```python
from build123d import *

# Parameters (mm, degrees)
F1_DEPTH = 2


with BuildPart() as f1:
    # F0 (on Top) → F1 (new body)
    with BuildSketch(Plane.XY):
        Polygon((0, 10), (0, 0), (10, 0), (300, 0), (300, 10), (10, 10), (10, 300), (0, 300), align=None)
        Polygon((7, 297), (7, 7), (297, 7), (297, 3), (3, 3), (3, 297), align=None, mode=Mode.SUBTRACT)
    extrude(amount=F1_DEPTH)


solid = f1.part
```
CAD build for the part. Positions are in the model's coordinates, mm. Coordinates: 2 decimals unless noted, no trailing zeros. Order: outer loops, then holes, each group sorted by start corner. A loop starts at its lowest first (then second) coordinate and runs counter-clockwise, first axis right, second up.
(1) Saw through at A-A, the plane x = 202. Write the cut outline in (y, z), and give its area (3 significant figures).
Solution:
outline: (0, 0) - (3, 0) - (3, 2) - (0, 2) - close; (7, 0) - (10, 0) - (10, 2) - (7, 2) - close
area: 12.0 mm2
(2) Drill centre line: L1, parallel to X at y = 214, z = 0.35. Where is it in solid material? Low to high.
Solution:
L1: x = 0 to 3, 7 to 10
(3) Pin check, flat tip, straight feed: pin 1 Ø1 at (x, z) = (111.5, 1.5) entering from +Y. Stop position of the tip, or through.
Solution:
pin 1: stops at y = 10
(4) Saw through at C-C, the plane z = 0.45. Write the cut outline in (x, y).
Solution:
outline: (0, 0) - (300, 0) - (300, 10) - (10, 10) - (10, 300) - (0, 300) - close; hole (3, 3) - (297, 3) - (297, 7) - (7, 7) - (7, 297) - (3, 297) - close
